Here's how the part is built. I have some questions about the finished solid (model axes, mm). A direction names the side the tool comes from. Round coordinates to 2 decimals unless told otherwise and drop trailing zeros. Order: outer loops, then holes, each group sorted by start corner. A loop starts at its lowest first (then second) coordinate and runs counter-clockwise, first axis right, second up. Notation, with made-up numbers: (-22.75, 31.5) -> (24.25, 31.5) arc R19 cw to (24.25, 46.5) -> close; hole circle Ø9 at (16.25, 63). An arc over 180 degrees is marked (long way). Use a Markdown table: item, result. Add a question column.
from build123d import *

# Parameters (mm, degrees)
BOSS_EXTRUDE1_DEPTH = 3
SKETCH4_W           = 12.125
SKETCH4_H           = 3.2
SKETCH4_W_2         = 4.8
SKETCH4_H_2         = 23.2
SKETCH4_W_3         = 2.7
CUT_EXTRUDE1_DEPTH  = 4


with BuildPart() as part:
    # Sketch1 → Boss-Extrude1 (new body)
    with BuildSketch(Plane(origin=(0, 0, 0), x_dir=(1, 0, 0), z_dir=(0, 1, 0))):
        with BuildLine():
            Line((37.95, 21.5), (28.05, 21.5))
            Line((28.05, 21.5), (28.05, 29.157009142))
            ThreePointArc((28.05, 29.157009142), (27.171320344, 31.278329486), (25.05, 32.157009142))
            Line((25.05, 32.157009142), (21.058452488, 32.157009142))
            Line((21.058452488, 32.157009142), (17.188733854, 30.83348742))
            Line((17.188733854, 30.83348742), (17.188733854, 29.16651258))
            Line((17.188733854, 29.16651258), (21.058452488, 27.842990858))
            Line((21.058452488, 27.842990858), (21.058452488, 26.157009142))
            Line((21.058452488, 26.157009142), (17.188733854, 24.83348742))
            Line((17.188733854, 24.83348742), (17.188733854, 23.16651258))
            Line((17.188733854, 23.16651258), (21.058452488, 21.842990858))
            Line((21.058452488, 21.842990858), (21.058452488, 20.157009142))
            Line((21.058452488, 20.157009142), (17.188733854, 18.83348742))
            Line((17.188733854, 18.83348742), (17.188733854, 17.16651258))
            Line((17.188733854, 17.16651258), (21.058452488, 15.842990858))
            Line((21.058452488, 15.842990858), (21.058452488, 14.157009142))
            Line((21.058452488, 14.157009142), (17.188733854, 12.83348742))
            Line((17.188733854, 12.83348742), (17.188733854, 11.16651258))
            Line((17.188733854, 11.16651258), (21.058452488, 9.842990858))
            Line((21.058452488, 9.842990858), (21.058452488, 8.157009142))
            Line((21.058452488, 8.157009142), (17.188733854, 6.83348742))
            Line((17.188733854, 6.83348742), (17.188733854, 5.16651258))
            Line((17.188733854, 5.16651258), (21.058452488, 3.842990858))
            Line((21.058452488, 3.842990858), (21.058452488, 2.157009142))
            Line((21.058452488, 2.157009142), (17.188733854, 0.83348742))
            Line((17.188733854, 0.83348742), (17.188733854, -0.83348742))
            Line((17.188733854, -0.83348742), (21.058452488, -2.157009142))
            Line((21.058452488, -2.157009142), (21.058452488, -3.842990858))
            Line((21.058452488, -3.842990858), (17.188733854, -5.16651258))
            Line((17.188733854, -5.16651258), (17.188733854, -6.83348742))
            Line((17.188733854, -6.83348742), (21.058452488, -8.157009142))
            Line((21.058452488, -8.157009142), (21.058452488, -9.842990858))
            Line((21.058452488, -9.842990858), (17.188733854, -11.16651258))
            Line((17.188733854, -11.16651258), (17.188733854, -12.83348742))
            Line((17.188733854, -12.83348742), (21.058452488, -14.157009142))
            Line((21.058452488, -14.157009142), (21.058452488, -15.842990858))
            Line((21.058452488, -15.842990858), (17.188733854, -17.16651258))
            Line((17.188733854, -17.16651258), (17.188733854, -18.83348742))
            Line((17.188733854, -18.83348742), (21.058452488, -20.157009142))
            Line((21.058452488, -20.157009142), (21.058452488, -21.842990858))
            Line((21.058452488, -21.842990858), (17.188733854, -23.16651258))
            Line((17.188733854, -23.16651258), (17.188733854, -24.83348742))
            Line((17.188733854, -24.83348742), (21.058452488, -26.157009142))
            Line((21.058452488, -26.157009142), (21.058452488, -27.842990858))
            Line((21.058452488, -27.842990858), (17.188733854, -29.16651258))
            Line((17.188733854, -29.16651258), (17.188733854, -30.83348742))
            Line((17.188733854, -30.83348742), (21.058452488, -32.157009142))
            Line((21.058452488, -32.157009142), (25.05, -32.157009142))
            ThreePointArc((25.05, -32.157009142), (27.171320344, -31.278329486), (28.05, -29.157009142))
            Line((28.05, -29.157009142), (28.05, -21.5))
            Line((28.05, -21.5), (37.95, -21.5))
            Line((37.95, -21.5), (37.95, -8.3))
            Line((37.95, -8.3), (29, -8.3))
            Line((29, -8.3), (29, 0.7))
            Line((29, 0.7), (37.95, 0.7))
            Line((37.95, 0.7), (37.95, 21.5))
        make_face()
    extrude(amount=-BOSS_EXTRUDE1_DEPTH)

    # Sketch4 → Cut-Extrude1 (cut, through all)
    with BuildSketch(Plane(origin=(0, 0, 0), x_dir=(1, 0, 0), z_dir=(0, 1, 0))):
        with Locations((31.9875, -20)):
            Rectangle(SKETCH4_W, SKETCH4_H)
        with Locations((35.65, -1.9)):
            Rectangle(SKETCH4_W_2, SKETCH4_H_2)
        with Locations((31.9875, 20)):
            Rectangle(SKETCH4_W, SKETCH4_H)
        with Locations((27.75, -3.8)):
            Rectangle(SKETCH4_W_3, SKETCH4_H)
    extrude(amount=-CUT_EXTRUDE1_DEPTH, mode=Mode.SUBTRACT)


solid = part.part
(1) I want a section at B-B on x = 36.25. List the corners of the cut face in (y, z) for me.
(2) Please list where these lines run through material, in increasing order: probe 1 along Z at (x, y) = (33, -0.7); probe 2 along Z at (x, y) = (26, -1); probe 3 along Z at (x, y) = (34, -1.4). Write a range as from..to.
(3) I want a section at D-D on x = 20.25. State how many separate pieces and enclosed holes the cut face has, and give its area (3 significant figures).
(4) I want a section at A-A on x = 30. List the corners of the cut face in (y, z) for me, and give its area (3 significant figures).
(5) I want a section at C-C on z = -15. List the corners of the cut face in (x, y) for me, and give its area (3 significant figures).
(6) I'm going to push flat-ended pins straight in: P1, Ø1.5, axis at y = -1.5, z = 4, coming from the +X side; P2, Ø1.5, axis at x = 36.5, y = -1.5, coming from the +Z side; P3, Ø1.3, axis at y = -1, z = -9, coming from the -X side; P4, Ø1, axis at x = 23, z = -3, coming from the +Y side. Where does each tip first touch, or does it pass through?
(7) On a 3-axis mill with a long thin cutter (end or side, diameter ignored), from which of +Z, -Z, +X, -X, +Y, -Y can I reach the whole of each face in a straight line? I mean faces 5 (the flat face through (17.189, -1, -6)), 6 (the flat face through (36, -1, 13.5)), 7 (the flat face through (21.058, -1, 27)). Say none if no direction works.
(8) If we mould it in two halves opening along Z, with no side actions, what happens to faces 1 (the flat face through (17.189, -1, -24)), 2 (the flat face through (19.151, -1.479, -31.505)), 3 (the flat face through (25.925, -1, 20)), 4 (the flat face through (21.058, -1, 15))? For each: pulls with the +Z half, pulls with the -Z half, needs draft (parallel to the pull), parting line crosses it, or undercut.
Output:
| question | item | result |
|---|---|---|
| 1 | outline | (-3, -18.4) -> (0, -18.4) -> (0, -9.7) -> (-3, -9.7) -> close; (-3, 13.5) -> (0, 13.5) -> (0, 18.4) -> (-3, 18.4) -> close |
| 2 | probe 1 | -18.4..-0.7, 8.3..18.4 |
| 2 | probe 2 | -32..-21.6, -18.4..18.4, 21.6..32 |
| 2 | probe 3 | -18.4..-9.7, 13.5..18.4 |
| 3 | separate pieces | 11 |
| 3 | enclosed holes | 0 |
| 3 | area | 124 mm² |
| 4 | outline | (-3, -18.4) -> (0, -18.4) -> (0, -0.7) -> (-3, -0.7) -> close; (-3, 8.3) -> (0, 8.3) -> (0, 18.4) -> (-3, 18.4) -> close |
| 4 | area | 83.4 mm² |
| 5 | outline | (21.06, -3) -> (37.95, -3) -> (37.95, 0) -> (21.06, 0) -> close |
| 5 | area | 50.7 mm² |
| 6 | P1 | x = 26.4 |
| 6 | P2 | z = 18.4 |
| 6 | P3 | x = 21.06 |
| 6 | P4 | y = 0 |
| 7 | face 5 | +Z, -Z, -X, +Y, -Y |
| 7 | face 6 | +X, +Y, -Y |
| 7 | face 7 | -X, +Y, -Y |
| 8 | face 1 | needs draft |
| 8 | face 2 | pulls with the -Z half |
| 8 | face 3 | undercut |
| 8 | face 4 | undercut |
